Autodesk Inventor part; units mm, degrees
ref_plane "YZ Plane" through (0, 0, 0) normal (1, 0, 0) x (0, 1, 0)
ref_plane "XZ Plane" through (0, 0, 0) normal (0, 1, 0) x (-1, 0, 0)
ref_plane "XY Plane" through (0, 0, 0) normal (0, 0, 1) x (1, 0, 0)
sketch "Sketch1" plane through (0, 0, 0) normal (0, 0, 1) x (1, 0, 0)
  line L0 (0, 28) -> (0, -28) construction
  line L1 (-28, 0) -> (28, 0) construction
  line L2 (-20, 20) -> (20, 20)
  line L3 (20, 20) -> (20, -20)
  line L4 (20, -20) -> (-20, -20)
  line L5 (-20, -20) -> (-20, 20)
  point P0 (0, 0)
  dimension "d0" = 40
  dimension "d1" = 40
extrude "Extrusion1" add sketch "Sketch1" along normal blind 20
sketch "Sketch4" plane through (0, 0, 20) normal (0, 0, 1) x (1, 0, 0)
  line L0 (-28, 0) -> (28, 0) construction
  line L1 (0, 28) -> (0, -28) construction
  line L2 (-12.6, 12.6) -> (12.6, 12.6) construction
  line L3 (12.6, 12.6) -> (12.6, -12.6) construction
  line L4 (12.6, -12.6) -> (-12.6, -12.6) construction
  line L5 (-12.6, -12.6) -> (-12.6, 12.6) construction
  point P0 (0, 0)
  dimension "d15" = 25.2
  dimension "d16" = 25.2
hole "Hole2" at (-12.6, 12.6, 20) at (12.6, 12.6, 20) at (12.6, -12.6, 20) at (-12.6, -12.6, 20) at (-12.6, 12.6, 20) at (12.6, 12.6, 20) direction (0, 0, -1) diameter 5 depth 8
sketch "Sketch5" plane through (0, 0, 20) normal (0, 0, 1) x (1, 0, 0)
  circle A0 centre (-12.6, 12.6) radius 2.5
  circle A1 centre (12.6, -12.6) radius 2.5
  line L0 (-12.6, 12.6) -> (12.6, 12.6)
  line L1 (12.6, 12.6) -> (12.6, -12.6)
  line L2 (12.6, -12.6) -> (-12.6, -12.6)
  line L3 (-12.6, -12.6) -> (-12.6, 12.6)
  point P0 (0, 0)
extrude "Extrusion3" cut sketch "Sketch5" against normal blind 8 contours L0 L1 A1 L2 L3 A0 | A0 L3 L0 | L1 L2 A1 picked at (-10.9542, 12.4146) picked at (11.1977, -11.7189)
sketch "Sketch6" plane through (-20, -20, 0) normal (-1, 0, 0) x (0, 0, 1)
  line L0 (0, 40) -> (20, 40)
  line L1 (20, 9.9) -> (12, 9.9) construction
  line L2 (20, 30.1) -> (20, 9.9) construction
  line L3 (12, 30.1) -> (20, 30.1) construction
  line L4 (12, 9.9) -> (12, 30.1) construction
  line L5 (16, 30.1) -> (16, 9.9) construction
  point P0 (0, 20)
  point P1 (16, 20)
  dimension "d27" = 20
hole "Hole3" at (-20, 0, 16) direction (1, 0, 0) diameter 3.242 end up to surface
sketch "Sketch8" plane through (0, 0, 0) normal (0, 0, -1) x (-1, 0, 0)
  line L0 (20, 20) -> (-20, 20) construction
  line L1 (-20, 20) -> (-20, -20) construction
  line L2 (-20, -20) -> (20, -20) construction
  line L3 (20, -20) -> (20, 20) construction
  line L4 (0, -31.5) -> (0, 31.5) construction
  line L5 (-28, 0) -> (28, 0) construction
  line L6 (-12.5, -12.5) -> (12.5, -12.5)
  line L7 (12.5, -12.5) -> (12.5, 12.5)
  line L8 (12.5, 12.5) -> (-12.5, 12.5)
  line L9 (-12.5, 12.5) -> (-12.5, -12.5)
  point P0 (0, 0)
  dimension "d44" = 25
  dimension "d45" = 25
extrude "Extrusion4" cut sketch "Sketch8" against normal blind 6
sketch "Sketch9" plane through (0, 0, 0) normal (0, 0, -1) x (-1, 0, 0)
  line L0 (12.5, 12.5) -> (12.5, -12.5) construction
  line L1 (12.5, -12.5) -> (-12.5, -12.5) construction
  line L2 (-12.5, -12.5) -> (-12.5, 12.5) construction
  line L3 (-12.5, 12.5) -> (12.5, 12.5) construction
  line L4 (20, 20) -> (-20, 20) construction
  line L5 (-20, 20) -> (-20, -20) construction
  line L6 (-20, -20) -> (20, -20) construction
  line L7 (20, -20) -> (20, 20) construction
  line L8 (12.5, -12.5) -> (-12.5, -12.5) construction
  point P0 (0, 0)
hole "Hole5" at (-12.5, 12.5, 0) at (-12.5, -12.5, 0) at (12.5, -12.5, 0) at (12.5, 12.5, 0) direction (0, 0, 1) diameter 3 depth 6
sketch "Sketch10" plane through (0, 0, 6) normal (0, 0, -1) x (-1, 0, 0)
  point P0 (0, 0)
  point P1 (0, 0)
hole "Hole6" at (0, 0, 6) direction (0, 0, 1) diameter 3.242 depth 4 tip angle 118
properties part number "Large-cuvette-mount-25mm-V3" material "PC/ABS Plastic"
For this review, take the finished solid that the model builds, in its own axes (mm). A direction names the side the tool comes from. Round coordinates to 2 decimals unless told otherwise and drop trailing zeros. Loops run counter-clockwise (first coordinate to the right, second up) from the corner with the lowest first, then second, coordinate; pieces in that order, holes last. Notation, with made-up numbers: (-10, 9) - (22, 9) arc R25 ccw to (22, 37) - close; hole circle Ø6 at (47.25, -25). An arc over 180 degrees is marked (long way). One line per question, with ' | ' between items.
Q1. For line 1 along X through (y, z) = (0, 7.1); line 2 along Y through (x, z) = (-9, 2.75), list the stretches that pass through material, from the lowest coordinate up. Write a range as [from, to].
Taken from the geometry:
line 1: x = [-20, -1.62], [1.62, 20] | line 2: y = [-20, -12.5], [12.5, 20]
Q2. Take a section at D-D (z = 16). Give the boundary of the cut face in (x, y), and give its area (3 significant figures).
Taken from the geometry:
outline: (-20, -20) - (20, -20) - (20, 20) - (-20, 20) - (-20, 1.62) - (-12.6, 1.62) - (-12.6, 10.1) arc R2.5 cw (long way) to (-10.1, 12.6) - (10.1, 12.6) arc R2.5 cw (long way) to (12.6, 10.1) - (12.6, -10.1) arc R2.5 cw (long way) to (10.1, -12.6) - (-10.1, -12.6) arc R2.5 cw (long way) to (-12.6, -10.1) - (-12.6, -1.62) - (-20, -1.62) - close | area: 882 mm²
Q3. Tool access review of faces 1 (the flat face through (3, 0, 6)), 2 (the flat face through (0, 20, 10)), 3 (the cylindrical face through (-14.309, -14.425, 15.944)): name each direction out of +Z, -Z, +X, -X, +Y, -Y from which nothing blocks a thin tool from reaching the whole face with its end or side.
Taken from the geometry:
face 1: -Z | face 2: +Z, -Z, +X, -X, +Y | face 3: +Z
Q4. The part is to be moulded in two halves that separate along X. For faces 4 (the flat face through (0, 14, 0)), 5 (the flat face through (-20, 0, 10)), 6 (the flat face through (0, -12.6, 16)), say which applies: released by +X, released by -X, zero draft, split by the parting line, or undercut.
Taken from the geometry:
face 4: zero draft | face 5: released by -X | face 6: undercut
Q5. Take a section at B-B (y = 3). Give the boundary of the cut face in (x, z), and give its area (3 significant figures).
Taken from the geometry:
outline: (-20, 0) - (-12.5, 0) - (-12.5, 6) - (12.5, 6) - (12.5, 0) - (20, 0) - (20, 20) - (12.6, 20) - (12.6, 12) - (-12.6, 12) - (-12.6, 20) - (-20, 20) - close | area: 448 mm²
Q6. For pin 1 (4 mm diameter, centred on x = -12.6, y = -12.6, fed in from +Z); pin 2 (2.5 mm diameter, centred on x = -12.5, y = -12.5, fed in from -Z), all flat-tipped, find the tip position at first contact; note any pin that passes through.
Taken from the geometry:
pin 1: stops at z = 12 | pin 2: stops at z = 6
